from build123d import *

# Parameters (mm, degrees)
SKETCH1_R           = 1.5
BOSS_EXTRUDE1_DEPTH = 3
SKETCH2_R           = 3.6
SKETCH2_R_2         = 2.9
BOSS_EXTRUDE2_DEPTH = 4.5


with BuildPart() as part:
    # Sketch1 → Boss-Extrude1 (new body)
    with BuildSketch(Plane(origin=(0, 0, 0), x_dir=(1, 0, 0), z_dir=(0, 1, 0))):
        Polygon((-6, 17), (-3, 20), (3, 20), (6, 17), (6, -17), (3, -20), (-3, -20), (-6, -17), align=None)
        with Locations(Location((0, 14, 0), (0, 0, 270))):
            Circle(SKETCH1_R, mode=Mode.SUBTRACT)
        with Locations(Location((0, -14, 0), (0, 0, 270))):
            Circle(SKETCH1_R, mode=Mode.SUBTRACT)
    extrude(amount=BOSS_EXTRUDE1_DEPTH)

    # Sketch2 → Boss-Extrude2 (add)
    with BuildSketch(Plane(origin=(0, 3, 0), x_dir=(1, 0, 0), z_dir=(0, 1, 0))):
        with Locations(Location((0, 14, 0), (0, 0, 270))):
            Circle(SKETCH2_R)
        with Locations(Location((0, 14, 0), (0, 0, 270))):
            Circle(SKETCH2_R_2, mode=Mode.SUBTRACT)
    extrude(amount=BOSS_EXTRUDE2_DEPTH)


solid = part.part
Geometry: final body of the model. Coordinates: model frame, mm. A direction names the side the tool comes from. Round coordinates to 2 decimals unless told otherwise and drop trailing zeros. Loops run counter-clockwise (first coordinate to the right, second up) from the corner with the lowest first, then second, coordinate; pieces in that order, holes last. Notation, with made-up numbers: M 88,68.5 L 109,68.5 A31 cw 109,101.5 Z; hole C 70,67 d2. An arc over 180 degrees is marked long. Put each result on its own line as item: value. Start each with the question number.
(1) Section query C-C (y = 2). Return loops of the section in (x, z).
(2) Set-up query: faces 1 (the face through (-1.2, 3, -12.8)), 2 (the face through (0.07, 1.48, -15.5)). Return all of +Z, -Z, +X, -X, +Y, -Y with unobstructed straight access to the full face (end or side cutting, diameter ignored); none if empty.
(3) Section query B-B (x = 0). Return loops of the section in (y, z), then the cut area to 3 significant figures.
(4) Material intervals for line 1 along X through (y, z) = (6.45, -14); line 2 along Y through (x, z) = (-5.5, -4.5); line 3 along Z through (x, y) = (-1, 2.75), sorted ascending. Write a range as [from, to].
(5) Draft query along X for faces 3 (the face through (0.07, 1.48, 12.5)), 4 (the face through (0, 0, 0)), 5 (the face through (0.158, 5.219, -17.597)). Return one class per face: +X half, -X half, draft (parallel to the pull), parting line (faces both ways), or undercut.
(6) Contact query for flat-ended pins moving along their axis: pin 1 Ø1 at (x, z) = (-0.5, -8.5) entering from +Y; pin 2 Ø1.5 at (x, y) = (1, 5) entering from +Z; pin 3 Ø1.8 at (x, z) = (0, 14) entering from +Y. Output: stop coordinate, or through.
(7) Section query A-A (z = 14). Return loops of the section in (x, y), then the cut area to 3 significant figures.
(8) Section query D-D (z = -14). Return loops of the section in (x, y).
Findings below:
1. outline: M -6,-17 L -3,-20 L 3,-20 L 6,-17 L 6,17 L 3,20 L -3,20 L -6,17 Z; hole C 0,-14 d3; hole C 0,14 d3
2. face 1: +Y
2. face 2: +Y, -Y
3. outline: M 0,-20 L 3,-20 L 3,-17.6 L 7.5,-17.6 L 7.5,-16.9 L 3,-16.9 L 3,-15.5 L 0,-15.5 Z; M 0,-12.5 L 3,-12.5 L 3,-11.1 L 7.5,-11.1 L 7.5,-10.4 L 3,-10.4 L 3,12.5 L 0,12.5 Z; M 0,15.5 L 3,15.5 L 3,20 L 0,20 Z
3. area: 108 mm2
4. line 1: x = [-3.6, -2.9], [2.9, 3.6]
4. line 2: y = [0, 3]
4. line 3: z = [-20, -15.12], [-12.88, 12.88], [15.12, 20]
5. face 3: undercut
5. face 4: draft
5. face 5: parting line
6. pin 1: stops at y = 3
6. pin 2: stops at z = -10.41
6. pin 3: passes through
7. outline: M -6,0 L -1.5,0 L -1.5,3 L -6,3 Z; M 1.5,0 L 6,0 L 6,3 L 1.5,3 Z
7. area: 27.0 mm2
8. outline: M -6,0 L -1.5,0 L -1.5,3 L -2.9,3 L -2.9,7.5 L -3.6,7.5 L -3.6,3 L -6,3 Z; M 1.5,0 L 6,0 L 6,3 L 3.6,3 L 3.6,7.5 L 2.9,7.5 L 2.9,3 L 1.5,3 Z
